Verification items for the finished model (mm, model axes). Coordinates: 2 decimals unless noted, no trailing zeros. Order: outer loops, then holes, each group sorted by start corner. A loop starts at its lowest first (then second) coordinate and runs counter-clockwise, first axis right, second up. Notation, with made-up numbers: M 49,-7.5 L 71,-7.5 A15 cw 71,7.5 Z; hole C -34,-3 d3. An arc over 180 degrees is marked long. Answer as a JSON object with one key per item and string values. Group by question number.
(1) Material ranges on line 1 (Y direction, x = 7, z = -13.25); line 2 (X direction, y = -23, z = -15); line 3 (X direction, y = -19, z = -13.9), recorded low to high.
(2) Gauge pin test, flat ends, axial feed: pin 1 Ø10 at (x, y) = (11.5, -12) entering from -Z; pin 2 Ø5 at (x, y) = (-7, -17.5) entering from +Z; pin 3 Ø5 at (x, y) = (19.5, -21.5) entering from +Z. Record the tip position at first contact, or that the pin passes through.
(3) Cross-section at A-A (z = -13.2). Enter the section's corners in (x, y).
(4) Cross-section at C-C (x = 13). Enter the section's corners in (y, z), plus the area to 3 significant figures.
(5) Cross-section at B-B (y = -19.05). Enter the section's corners in (x, z), plus the area to 3 significant figures.
(6) Cross-section at D-D (y = -27). Enter the section's corners in (x, z).
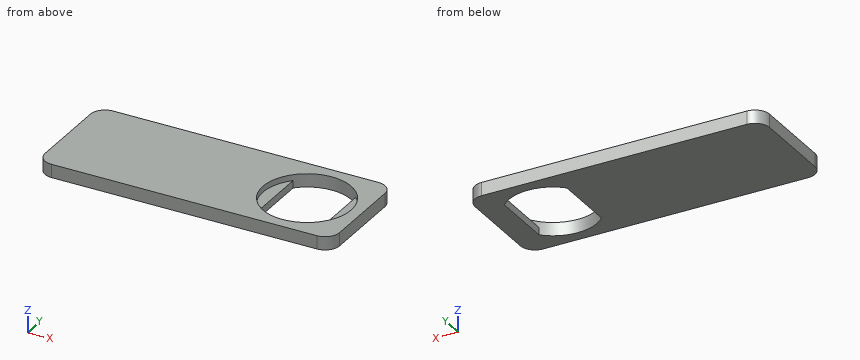
from build123d import *

# Parameters (mm, degrees)
F0_W     = 101.6
F0_H     = 4.572
F1_DEPTH = 38.1
F2_R     = 5.08
F4_D     = 30.48
F6_START = -2.032
F6_DEPTH = 2.54


with BuildPart() as f1:
    # F0 (on Front) → F1 (new body)
    with BuildSketch(Plane.XZ):
        with Locations((-24.6199596018, -14.7750445657)):
            Rectangle(F0_W, F0_H)
    extrude(amount=F1_DEPTH)

    # F2
    f2_edges = [f1.edges().sort_by_distance(p)[0] for p in [
        (26.18004, -38.1, -14.775045),
        (26.18004, 0, -14.775045),
        (-75.41996, -38.1, -14.775045),
        (-75.41996, 0, -14.775045),
    ]]
    fillet(f2_edges, radius=F2_R)

    # F4 (through all)
    with Locations(Plane.XY.offset(-12.4890445657)):
        with Locations((7.1300403982, -19.05)):
            Hole(F4_D / 2)

    # F5 (on face) → F6 (join)
    with BuildSketch(Plane.XY.offset(-12.4890445657).offset(F6_START)):
        with BuildLine():
            ThreePointArc((22.3700403982, -19.05), (21.2159885399, -13.2324691706), (17.9286145516, -8.2960055675))
            Line((17.9286145516, -8.2960055675), (17.9286145516, -29.8039944325))
            ThreePointArc((17.9286145516, -29.8039944325), (21.2159885399, -24.8675308294), (22.3700403982, -19.05))
        make_face()
        with BuildLine():
            Line((-3.6613854484, -29.8111676038), (-3.6613854484, -8.2888323962))
            ThreePointArc((-3.6613854484, -8.2888323962), (-8.1099596018, -19.05), (-3.6613854484, -29.8111676038))
        make_face()
    extrude(amount=-F6_DEPTH)


solid = f1.part
Taken from the geometry:
{
 "1": {"line 1": "y = -38.1 to -34.29, -3.81 to 0", "line 2": "x = -75.42 to -3.66, 17.93 to 26.18", "line 3": "x = -75.42 to -8.11, 22.37 to 26.18"},
 "2": {"pin 1": "passes through", "pin 2": "stops at z = -12.49", "pin 3": "stops at z = -14.52"},
 "3": {"outline": "M -75.42,-33.02 A5.08 ccw -70.34,-38.1 L 21.1,-38.1 A5.08 ccw 26.18,-33.02 L 26.18,-5.08 A5.08 ccw 21.1,0 L -70.34,0 A5.08 ccw -75.42,-5.08 Z; hole C 7.13,-19.05 d30.48"},
 "4": {"outline": "M -38.1,-17.06 L -33.11,-17.06 L -33.11,-12.49 L -38.1,-12.49 Z; M -4.99,-17.06 L 0,-17.06 L 0,-12.49 L -4.99,-12.49 Z", "area": "45.6 mm²"},
 "5": {"outline": "M -75.42,-17.06 L -3.66,-17.06 L -3.66,-14.52 L -8.11,-14.52 L -8.11,-12.49 L -75.42,-12.49 Z; M 17.93,-17.06 L 26.18,-17.06 L 26.18,-12.49 L 22.37,-12.49 L 22.37,-14.52 L 17.93,-14.52 Z", "area": "348 mm²"},
 "6": {"outline": "M -75.42,-17.06 L -3.66,-17.06 L -3.66,-14.52 L -5.87,-14.52 L -5.87,-12.49 L -75.42,-12.49 Z; M 17.93,-17.06 L 26.18,-17.06 L 26.18,-12.49 L 20.13,-12.49 L 20.13,-14.52 L 17.93,-14.52 Z"}
}
